from build123d import *

# Parameters (mm, degrees)
SKETCH1_W           = 3
SKETCH1_H           = 30.2
BOSS_EXTRUDE1_DEPTH = 3


with BuildPart() as part:
    # Sketch1 → Boss-Extrude1 (new body)
    with BuildSketch(Plane.XY):
        Polygon((247, 49.4), (0, 0), (25.1, 0), (25.1, 3), (49.9, 3), (49.9, 0), (75.1, 0), (75.1, 3), (99.9, 3), (99.9, 0), (125.1, 0), (125.1, 3), (149.9, 3), (149.9, 0), (175.1, 0), (175.1, 3), (199.9, 3), (199.9, 0), (225.1, 0), (225.1, 3), (247, 3), (247, 9.9), (247, 40.1), align=None)
        with Locations((248.5, 25)):
            Rectangle(SKETCH1_W, SKETCH1_H)
    extrude(amount=BOSS_EXTRUDE1_DEPTH)


solid = part.part
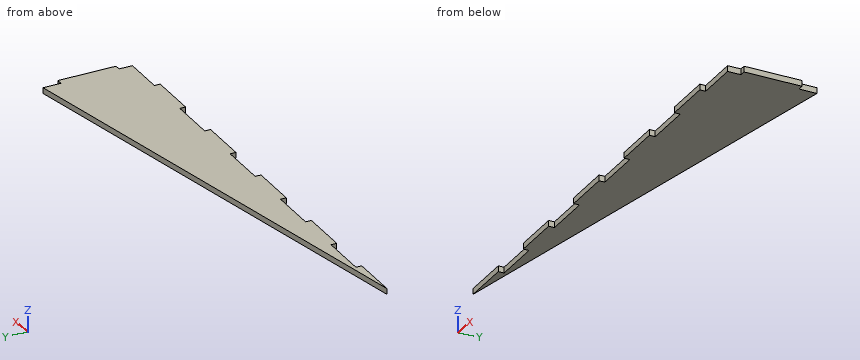
The listing builds one solid part. Answer for the finished solid, in the listing's coordinates (mm). Round coordinates to 2 decimals unless told otherwise and drop trailing zeros. Write each loop counter-clockwise with the first axis right and the second up, starting at its lowest first coordinate (ties: lowest second). Pieces come first, ordered by that corner, then holes. Notation, with made-up numbers: M -10.5,32 L 33.5,32 A21 ccw 33.5,68 Z; hole C -28,-12.75 d4. An arc over 180 degrees is marked long. Write each question's results on one line, items separated by ' | '. Start each with the question number.
Item 1: Find section C-C on x = 140. Write down the section's boundary in (y, z).
Item 2: Find section B-B on y = 21. Write down the section's boundary in (x, z).
Item 3: Given pin 1 Ø0.9 at (y, z) = (1.5, 1) entering from +X; pin 2 Ø1.5 at (x, z) = (132, 2) entering from -Y; pin 3 Ø1 at (x, z) = (215, 2) entering from +Y, each flat-ended and moving along its own axis, determine where each tip first touches the part or whether it passes through.
Item 4: Find section A-A on z = 1.5. Write down the section's boundary in (x, y), and give its area (3 significant figures).
Item 5: Straight lines are drawn through the part: probe 1 along Y at (x, z) = (36, 1.55); probe 2 along Y at (x, z) = (185.5, 2.2). For each, find the intervals that lie inside material, in ascending order.
Answer block:
1) outline: M 3,0 L 28,0 L 28,3 L 3,3 Z
2) outline: M 105,0 L 250,0 L 250,3 L 105,3 Z
3) pin 1: stops at x = 225.1 | pin 2: stops at y = 3 | pin 3: stops at y = 43.1
4) outline: M 0,0 L 25.1,0 L 25.1,3 L 49.9,3 L 49.9,0 L 75.1,0 L 75.1,3 L 99.9,3 L 99.9,0 L 125.1,0 L 125.1,3 L 149.9,3 L 149.9,0 L 175.1,0 L 175.1,3 L 199.9,3 L 199.9,0 L 225.1,0 L 225.1,3 L 247,3 L 247,9.9 L 250,9.9 L 250,40.1 L 247,40.1 L 247,49.4 Z | area: 5,830 mm²
5) probe 1: y = 3 to 7.2 | probe 2: y = 3 to 37.1
